Input: part model. Units: mm. Frame: model coordinates. Face numbers are marked on the shaded views. A direction names the side the tool comes from. Round coordinates to 2 decimals unless told otherwise and drop trailing zeros. Loops run counter-clockwise (first coordinate to the right, second up) from the corner with the lowest first, then second, coordinate; pieces in that order, holes last. Notation, with made-up numbers: M 78,56.25 L 124,56.25 A29 cw 124,94.25 Z; hole C 17.5,2.25 d7. An arc over 180 degrees is marked long. Put each result on its own line as item: value. Start each with the question number.
1) Section A-A on x = 0. Output: boundary loops of the cut face in (y, z), plus the area to 3 significant figures.
2) Section B-B on y = -5.5. Output: boundary loops of the cut face in (x, z), plus the area to 3 significant figures.
3) Section C-C on y = -12.5. Output: boundary loops of the cut face in (x, z).
4) Pin query (flat end, axial travel): pin 1 (3 mm diameter, centred on x = -18, z = 0, fed in from +Y); pin 2 (5.5 mm diameter, centred on x = 18, z = 0, fed in from +Y); pin 3 (4.5 mm diameter, centred on x = -18, z = 0, fed in from +Y). Return the tip coordinate at first contact, or that it passes through.
5) Draft query along Y for the marked faces 3, 4 and 5. Return one class per face: +Y half, -Y half, draft (parallel to the pull), parting line (faces both ways), or undercut.
6) Section D-D on z = -5.25. State how many separate pieces and enclosed holes the cut face has, plus the area to 3 significant figures.
7) Reachability of the marked faces 1 and 2 from +Z, -Z, +X, -X, +Y, -Y: full face, straight path, thin tool, end or side. Return the list, or none.
8) Line query: probe 1 along X at (y, z) = (0, -2.75); probe 2 along X at (y, z) = (21.75, 0). Output: solid intervals per line, ascending.
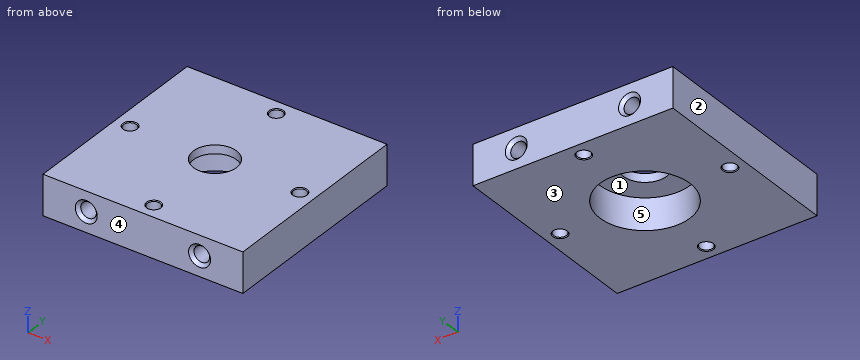
Autodesk Inventor part; units mm, degrees
ref_plane "YZ Plane" through (0, 0, 0) normal (1, 0, 0) x (0, 1, 0)
ref_plane "XZ Plane" through (0, 0, 0) normal (0, 1, 0) x (-1, 0, 0)
ref_plane "XY Plane" through (0, 0, 0) normal (0, 0, 1) x (1, 0, 0)
sketch "Sketch1" plane through (0, 0, 0) normal (0, 0, 1) x (1, 0, 0)
  line L0 (-31.75, 31.75) -> (31.75, 31.75)
  line L1 (31.75, 31.75) -> (31.75, -31.75)
  line L2 (31.75, -31.75) -> (-31.75, -31.75)
  line L3 (-31.75, -31.75) -> (-31.75, 31.75)
  line L4 (0, 0) -> (0, 31.75) construction
  line L5 (0, 0) -> (0, -31.75) construction
  line L6 (0, 0) -> (31.75, 0) construction
  line L7 (0, 0) -> (-31.75, 0) construction
  dimension "d0" = 63.5
  dimension "d1" = 63.5
extrude "Extrusion1" add sketch "Sketch1" along normal mid plane 12.7
sketch "Sketch9" plane through (-31.75, -31.75, 6.35) normal (0, -1, 0) x (1, 0, 0)
  line L0 (63.5, 0) -> (0, 0)
  line L1 (0, 0) -> (0, -12.7)
  line L2 (0, -12.7) -> (63.5, -12.7)
  line L3 (63.5, 0) -> (63.5, -12.7)
  line L4 (0, -6.35) -> (63.5, -6.35) construction
  line L5 (31.75, 0) -> (31.75, -12.7) construction
  point P0 (13.75, -6.35)
  dimension "d37" = 18
hole "Hole3" at (-18, -31.75, 0) direction (0, 1, 0) diameter 4.978 depth 13.7 tip angle 118
mirror "Mirror1" about plane through (0, 0, 0) normal (1, 0, 0) of "Hole3"
mirror "Mirror2" about plane through (0, 0, 0) normal (0, 1, 0) of "Hole3", "Mirror1"
chamfer "Chamfer2" distance 1 angle 45 4 edges at (-18, -31.75, 2.489) (18, -31.75, 2.489) (-18, 31.75, 2.489) (18, 31.75, 2.489)
sketch "Sketch12" plane through (0, 0, -6.35) normal (0, 0, -1) x (-1, 0, 0)
  point P0 (0, 0)
  point P1 (0, 0)
hole "Hole6" at (0, 0, -6.35) direction (0, 0, 1) diameter 13.7 end through all counterbore diameter 28.575 counterbore depth 10
sketch "Sketch11" plane through (0, 0, 6.35) normal (0, 0, 1) x (1, 0, 0)
  circle A0 centre (0, 0) radius 6.85
  line L0 (31.75, 31.75) -> (31.75, -31.75)
  line L1 (0, 0) -> (31.75, 0) construction
  point P0 (26.9875, 0)
  dimension "d82" = 26.9875
hole "Hole5" at (26.9875, 0, 6.35) direction (0, 0, -1) diameter 4.134 end through all
pattern_circular "Circular Pattern4" count 4 over 360 about axis through (0, 0, 84.3461) along (0, 0, -1) of "Hole5"
chamfer "Chamfer3" distance 0.25 angle 45 8 edges at (26.9875, 2.067, 6.35) (2.067, -26.9875, -6.35) (-26.9875, -2.067, -6.35) (-2.067, 26.9875, -6.35) (26.9875, 2.067, -6.35) (-2.067, 26.9875, 6.35) (-26.9875, -2.067, 6.35) (2.067, -26.9875, 6.35)
properties part number "BB2-FrontPlate" material "Aluminum-6061-AHC"
Geometry results:
1. outline: M -31.75,-6.35 L -29.3,-6.35 L -29.05,-6.1 L -29.05,6.1 L -29.3,6.35 L -31.75,6.35 Z; M -24.92,-6.1 L -24.67,-6.35 L -14.29,-6.35 L -14.29,3.65 L -6.85,3.65 L -6.85,6.35 L -24.67,6.35 L -24.92,6.1 Z; M 6.85,3.65 L 14.29,3.65 L 14.29,-6.35 L 24.67,-6.35 L 24.92,-6.1 L 24.92,6.1 L 24.67,6.35 L 6.85,6.35 Z; M 29.05,-6.1 L 29.3,-6.35 L 31.75,-6.35 L 31.75,6.35 L 29.3,6.35 L 29.05,6.1 Z
1. area: 378 mm²
2. outline: M -31.75,-6.35 L -13.19,-6.35 L -13.19,3.65 L -4.08,3.65 L -4.08,6.35 L -31.75,6.35 Z; M 4.08,3.65 L 13.19,3.65 L 13.19,-6.35 L 31.75,-6.35 L 31.75,6.35 L 4.08,6.35 Z
2. area: 521 mm²
3. outline: M -31.75,-6.35 L -6.92,-6.35 L -6.92,3.65 L 6.92,3.65 L 6.92,-6.35 L 31.75,-6.35 L 31.75,6.35 L -31.75,6.35 Z
4. pin 1: stops at y = 17.46
4. pin 2: stops at y = 31.01
4. pin 3: stops at y = 17.91
5. face 3: draft
5. face 4: -Y half
5. face 5: undercut
6. separate pieces: 1
6. enclosed holes: 5
6. area: 3,340 mm²
7. face 1: -Z
7. face 2: +Z, -Z, -X, +Y, -Y
8. probe 1: x = -31.75 to -29.05, -24.92 to -14.29, 14.29 to 24.92, 29.05 to 31.75
8. probe 2: x = -31.75 to -20.49, -15.51 to 15.51, 20.49 to 31.75
